Autodesk Inventor part; units mm, degrees
ref_plane "YZ Plane" through (0, 0, 0) normal (1, 0, 0) x (0, 1, 0)
ref_plane "XZ Plane" through (0, 0, 0) normal (0, 1, 0) x (-1, 0, 0)
ref_plane "XY Plane" through (0, 0, 0) normal (0, 0, 1) x (1, 0, 0)
sketch "Sketch1" plane through (0, 0, 0) normal (0, 1, 0) x (-1, 0, 0)
  line L0 (0, 0) -> (0, -12)
  line L1 (0, -12) -> (38.1, -12)
  line L2 (38.1, -12) -> (38.1, 0)
  line L3 (38.1, 0) -> (0, 0)
  circle A0 centre (6.35, -6) radius 1.6256
  circle A1 centre (31.75, -6) radius 1.6256
  point P0 (0, -6)
  dimension "d0" = 3.2512
  dimension "d1" = 3.2512
  dimension "d3" = 0
  dimension "d4" = 12
  dimension "d6" = 38.1
  dimension "d37" = 6.35
  dimension "d38" = 6.35
extrude "Extrusion1" add sketch "Sketch1" along normal blind 6 contours L3 L2 L1 L0 | A0 | A1
sketch "Sketch3" plane through (0, 6, 0) normal (0, 1, 0) x (1, 0, 0)
  line L0 (-14.05, 0) -> (-24.05, 0)
  line L1 (-24.05, 0) -> (-24.05, 12)
  line L2 (-24.05, 12) -> (-14.05, 12)
  line L3 (-14.05, 12) -> (-14.05, 0)
  line L4 (-38.1, 0) -> (0, 0)
  line L5 (0, 0) -> (0, 12)
  line L6 (0, 12) -> (-38.1, 12)
  point P0 (-19.05, 12)
  point P1 (-19.05, 12)
  point P2 (-19.05, 12)
  dimension "d12" = 10
  dimension "d14" = 0
extrude "Extrusion3" add sketch "Sketch3" along normal blind 24.13 contours L0 L1 L2 L3
chamfer "Chamfer1" distance 3 angle 45 2 edges at (-14.05, 6, -6) (-24.05, 6, -6)
sketch "Sketch5" plane through (0, 30.13, 0) normal (0, 1, 0) x (1, 0, 0)
  line L0 (-14.05, 12) -> (-24.05, 12)
  line L1 (-14.05, 0) -> (-14.05, 12)
  point P0 (0, 0)
  point P1 (-19.05, 6)
  point P2 (-19.05, 12)
  point P3 (-14.05, 6)
hole "Hole1" at (-19.05, 30.13, -6) direction (0, -1, 0) diameter 4.7 end through all
hole "Hole2" at (-6.35, 0, -6) at (-31.75, 0, -6) direction (0, 1, 0) diameter 4.5 end through all
sketch "Sketch7" plane through (0, 30.13, 0) normal (0, 1, 0) x (1, 0, 0)
  line L0 (-14.05, 12) -> (-24.05, 12)
  line L1 (-24.05, 12) -> (-24.05, 14)
  line L2 (-24.05, 14) -> (-14.05, 14)
  line L3 (-11.05, 12) -> (-14.05, 12)
  line L4 (-24.05, 12) -> (-14.05, 12)
  line L5 (-14.05, 0) -> (-14.05, 12)
  line L6 (-14.05, 0) -> (-14.05, -2)
  line L7 (-14.05, -2) -> (-24.05, -2)
  line L8 (-24.05, 0) -> (-14.05, 0)
  line L9 (-24.05, -2) -> (-24.05, 0)
  line L10 (-24.05, 0) -> (-14.05, 0)
  line L11 (-24.05, 14) -> (-26.05, 14)
  line L12 (-26.05, 14) -> (-26.05, -2)
  line L13 (-26.05, -2) -> (-24.05, -2)
  line L14 (-24.05, -2) -> (-24.05, 14)
  line L15 (-14.05, -2) -> (-12.05, -2)
  line L16 (-12.05, -2) -> (-12.05, 14)
  line L17 (-12.05, 14) -> (-14.05, 14)
  line L18 (-14.05, 12) -> (-14.05, -2)
  point P0 (0, 0)
  point P1 (-12.05, 12)
  point P2 (-24.05, 0)
  point P3 (-25.05, -2)
  dimension "d41" = 2
  dimension "d42" = 2
  dimension "d43" = 2
  dimension "d44" = 2
extrude "Extrusion6" add sketch "Sketch7" against normal up to surface (30.13 mm away) contours L0 L1 L2 L17 L16 L3 | L3 L16 L15 L6 L5 | L14 L9 L13 L12 L11 L1 | L6 L7 L9 L8
sketch "Sketch6" plane through (0, 30.13, 0) normal (0, 1, 0) x (1, 0, 0)
  line L0 (-17.0293, 9.5) -> (-16.0189, 7.75)
  line L1 (-16.0189, 7.75) -> (-15.0085, 6)
  line L2 (-15.0085, 6) -> (-16.0189, 4.25)
  line L3 (-16.0189, 4.25) -> (-17.0293, 2.5)
  line L4 (-17.0293, 2.5) -> (-19.05, 2.5)
  line L5 (-19.05, 2.5) -> (-21.0707, 2.5)
  line L6 (-21.0707, 2.5) -> (-22.0811, 4.25)
  line L7 (-22.0811, 4.25) -> (-23.0915, 6)
  line L8 (-23.0915, 6) -> (-22.0811, 7.75)
  line L9 (-22.0811, 7.75) -> (-21.0707, 9.5)
  line L10 (-21.0707, 9.5) -> (-19.05, 9.5)
  line L11 (-19.05, 9.5) -> (-17.0293, 9.5)
  line L12 (-19.05, 10.3656) -> (-21.5705, 10.3656)
  line L13 (-16.5295, 10.3656) -> (-19.05, 10.3656)
  line L14 (-15.2693, 8.1828) -> (-16.5295, 10.3656)
  line L15 (-14.009, 6) -> (-15.2693, 8.1828)
  line L16 (-15.2693, 3.8172) -> (-14.009, 6)
  line L17 (-16.5295, 1.6344) -> (-15.2693, 3.8172)
  line L18 (-19.05, 1.6344) -> (-16.5295, 1.6344)
  line L19 (-21.5705, 1.6344) -> (-19.05, 1.6344)
  line L20 (-22.8307, 3.8172) -> (-21.5705, 1.6344)
  line L21 (-24.091, 6) -> (-22.8307, 3.8172)
  line L22 (-22.8307, 8.1828) -> (-24.091, 6)
  line L23 (-21.5705, 10.3656) -> (-22.8307, 8.1828)
  line L24 (-21.6282, 10.4656) -> (-16.4718, 10.4656)
  line L25 (-16.4718, 10.4656) -> (-13.8935, 6)
  line L26 (-13.8935, 6) -> (-16.4718, 1.5344)
  line L27 (-16.4718, 1.5344) -> (-21.6282, 1.5344)
  line L28 (-21.6282, 1.5344) -> (-24.2065, 6)
  line L29 (-24.2065, 6) -> (-21.6282, 10.4656)
  point P0 (0, 0)
  dimension "d50" = 0.1
  dimension "d51" = 0.1
  dimension "d52" = 0.1
  dimension "d53" = 0.1
  dimension "d54" = 0.1
  dimension "d55" = 0.1
extrude "Extrusion5" cut sketch "Sketch6" against normal blind 3.2 contours L0 L1 L2 L3 L4 L5 L6 L7 L8 L9 L10 L11 | L13 L14 L15 L16 L17 L18 L19 L20 L21 L22 L23 L12 | L24 L25 L26 L27 L28 L29
fillet "Fillet1" radius 2 4 edges at (-12.05, 15.065, -14) (-26.05, 15.065, -14) (-26.05, 15.065, 2) (-12.05, 15.065, 2)
properties part number "Hopper Rest Metric Wide"
For this review, take the finished solid that the model builds, in its own axes (mm). A direction names the side the tool comes from. Round coordinates to 2 decimals unless told otherwise and drop trailing zeros. Write each loop counter-clockwise with the first axis right and the second up, starting at its lowest first coordinate (ties: lowest second). Pieces come first, ordered by that corner, then holes. Notation, with made-up numbers: M -19,65.5 L 4,65.5 A27 cw 4,101.5 Z; hole C 42,-24.5 d11. An arc over 180 degrees is marked long. One line per item, written item: value. Start each with the question number.
(1) Machinability: for faces 4 (the flat face through (-6, 3, -12)), 5 (the flat face through (-4, 6, -5)), 6 (the flat face through (-15.165, 28.552, -3.798)), which of the approach directions +Z, -Z, +X, -X, +Y, -Y give a long, thin tool a straight path to every point of the face, cutting with its end or side? Answer none if there is none.
(2) We need section B-B (y = 3.5). Give the boundary of the cut face in (x, z), and give its area (3 significant figures).
(3) Insertion check: pin 1 (4 mm diameter, centred on y = 17.5, z = -2.5, fed in from +X); pin 2 (3.5 mm diameter, centred on x = -35, z = -6, fed in from +Y); pin 3 (4 mm diameter, centred on x = -6.35, z = -6, fed in from +Y); pin 4 (2 mm diameter, centred on x = -4, y = 3.5, fed in from +Z). Each pin has a flat end and moves straight along its axis. Give the tip position at first contact, or say it passes through.
(4) We need section D-D (x = -19.05). Give the boundary of the cut face in (y, z), and give its area (3 significant figures).
(5) The part is to be moulded in two halves that separate along Z. For faces 1 (the flat face through (-34, 6, -5)), 2 (the flat face through (-22.9, 28.55, -3.74)), 3 (the cylindrical face through (-25.48, 14.85, -13.4)), say which applies: released by +Z, released by -Z, zero draft, split by the parting line, or undercut.
(6) We need section C-C (y = 21). Give the boundary of the cut face in (x, z).
(7) Wall thickness on line 1 (X direction, y = 1.3, z = -6); line 2 (X direction, y = 10.5, z = -6); line 3 (Z direction, x = -31.75, y = 1.95): over which ranges is each line inside the solid? List them lowest first.
(8) We need section A-A (x = -6.35). Give the boundary of the cut face in (y, z), and give its area (3 significant figures).
Result:
1. face 4: -Z, +X, +Y, -Y
1. face 5: +Z, -Z, +X, +Y
1. face 6: +Y
2. outline: M -38.1,-12 L -26.05,-12 A2 ccw -24.05,-14 L -14.05,-14 A2 ccw -12.05,-12 L 0,-12 L 0,0 L -12.05,0 A2 ccw -14.05,2 L -24.05,2 A2 ccw -26.05,0 L -38.1,0 Z; hole C -31.75,-6 d4.5; hole C -19.05,-6 d4.7; hole C -6.35,-6 d4.5
2. area: 461 mm²
3. pin 1: x = -12.05
3. pin 2: y = 6
3. pin 3: through
3. pin 4: z = 0
4. outline: M 0,-14 L 30.13,-14 L 30.13,-10.47 L 26.93,-10.47 L 26.93,-8.35 L 0,-8.35 Z; M 0,-3.65 L 26.93,-3.65 L 26.93,-1.53 L 30.13,-1.53 L 30.13,2 L 0,2 Z
4. area: 327 mm²
5. face 1: zero draft
5. face 2: undercut
5. face 3: released by -Z
6. outline: M -26.05,-12 A2 ccw -24.05,-14 L -14.05,-14 A2 ccw -12.05,-12 L -12.05,0 A2 ccw -14.05,2 L -24.05,2 A2 ccw -26.05,0 Z; hole C -19.05,-6 d4.7
7. line 1: -38.1 to -34, -29.5 to -21.4, -16.7 to -8.6, -4.1 to 0
7. line 2: -26.05 to -21.4, -16.7 to -12.05
7. line 3: -12 to -8.25, -3.75 to 0
8. outline: M 0,-12 L 6,-12 L 6,-8.25 L 0,-8.25 Z; M 0,-3.75 L 6,-3.75 L 6,0 L 0,0 Z
8. area: 45.0 mm²
